```python
from build123d import *

# Parameters (mm, degrees)
FILLET1_R = 1


with BuildPart() as part:
    # Sketch1 → Revolve1 (revolve)
    with BuildSketch(Plane.XY, mode=Mode.PRIVATE) as revolve1_sk:
        Polygon((-21.5, 0), (-25, 0), (-25, 10), (-21.5, 10), (-21.5, 9), (-24, 9), (-24, 1), (-21.5, 1), align=None)
    revolve(revolve1_sk.sketch.rotate(Axis((0, 9.085123741, 0), (0, -1, 0)), 270), axis=Axis((0, 9.085123741, 0), (0, -1, 0)))

    # Fillet1
    fillet1_edges = [part.edges().sort_by_distance(p)[0] for p in [
        (0, 0, -25),
        (0, 10, -25),
    ]]
    fillet(fillet1_edges, radius=FILLET1_R)


solid = part.part
```
Build history of the part. All positions in model axes, mm. A direction names the side the tool comes from. Give positions to 0.01 mm unless a question says otherwise; leave off trailing zeros. Loops run counter-clockwise (first coordinate to the right, second up) from the corner with the lowest first, then second, coordinate; pieces in that order, holes last. Notation, with made-up numbers: (39, 3.25) -> (59, 3.25) arc R29 cw to (59, 42.25) -> close; hole circle Ø6 at (51.5, 26). An arc over 180 degrees is marked (long way). One line per question, with ' | ' between items.
Q1. Pull direction X, two halves, no side cores. Call faces 3 (the flat face through (-9, 0, 20)), 4 (the cylindrical face through (-7.509, 5.056, 23.846)), 5 (the cylindrical face through (-7.21, 4.94, 22.89)): pulls with the +X half, pulls with the -X half, needs draft (parallel to the pull), parting line crosses it, or undercut.
Filled sheet:
face 3: needs draft | face 4: parting line crosses it | face 5: undercut
Q2. Tool access for faces 1 (the flat face through (-9, 10, -20)), 2 (the flat face through (-9, 9, 20)): list every direction of +Z, -Z, +X, -X, +Y, -Y with a clear straight run to the whole face (end or side of a thin tool).
Filled sheet:
face 1: +Z, -Z, +X, -X, +Y | face 2: none
Q3. Drill centre lines: line 1 along Y through (x, z) = (18, 15.5); line 2 along X through (y, z) = (3, 0); line 3 along Z through (x, y) = (-11, 7.5). Where is each one in solid material? Low to high. Write a range as [from, to].
Filled sheet:
line 1: y = [0, 1], [9, 10] | line 2: x = [-25, -24], [24, 25] | line 3: z = [-22.45, -21.33], [21.33, 22.45]
Q4. Drop flat-ended pins along their axis: pin 1 (24 mm diameter, centred on x = 9, z = -12, fed in from +Y); pin 2 (2 mm diameter, centred on x = 5, y = 6.5, fed in from +Z); pin 3 (5 mm diameter, centred on y = 7, z = 17, fed in from -X); pin 4 (4 mm diameter, centred on y = 1.5, z = -20, fed in from -X). Give the stop position or say it passes through.
Filled sheet:
pin 1: stops at y = 10 | pin 2: stops at z = 24.68 | pin 3: stops at x = -20.37 | pin 4: stops at x = -17.35
Q5. Cut at A-A, the plane x = 0. Write the cut outline in (y, z), plus the area to 3 significant figures.
Filled sheet:
outline: (0, -24) arc R1 ccw to (1, -25) -> (9, -25) arc R1 ccw to (10, -24) -> (10, -21.5) -> (9, -21.5) -> (9, -24) -> (1, -24) -> (1, -21.5) -> (0, -21.5) -> close; (0, 21.5) -> (1, 21.5) -> (1, 24) -> (9, 24) -> (9, 21.5) -> (10, 21.5) -> (10, 24) arc R1 ccw to (9, 25) -> (1, 25) arc R1 ccw to (0, 24) -> close | area: 29.1 mm²
Q6. Cut at B-B, the plane z = 0. Write the cut outline in (x, y).
Filled sheet:
outline: (-25, 1) arc R1 ccw to (-24, 0) -> (-21.5, 0) -> (-21.5, 1) -> (-24, 1) -> (-24, 9) -> (-21.5, 9) -> (-21.5, 10) -> (-24, 10) arc R1 ccw to (-25, 9) -> close; (21.5, 0) -> (24, 0) arc R1 ccw to (25, 1) -> (25, 9) arc R1 ccw to (24, 10) -> (21.5, 10) -> (21.5, 9) -> (24, 9) -> (24, 1) -> (21.5, 1) -> close
